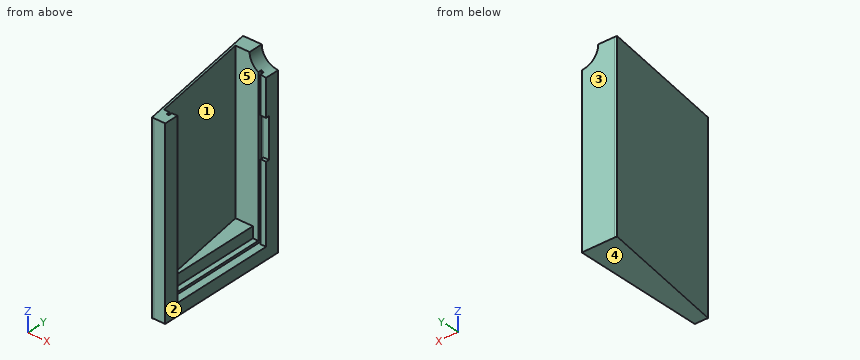
```python
from build123d import *

# Parameters (mm, degrees)
BOSS_EXTRUDE3_DEPTH = 40
SKETCH4_W           = 2
SKETCH4_H           = 142
CUT_EXTRUDE1_DEPTH  = 3
SKETCH5_W           = 2
SKETCH5_H           = 98
CUT_EXTRUDE2_DEPTH  = 3
SKETCH6_W           = 2
SKETCH6_H           = 145
CUT_EXTRUDE3_DEPTH  = 3
CUT_EXTRUDE4_DEPTH  = 228
SKETCH8_W           = 165
SKETCH8_H           = 122.641754717
BOSS_EXTRUDE5_DEPTH = 2
SKETCH11_W          = 2
SKETCH11_H          = 0.3
CUT_EXTRUDE5_DEPTH  = 145
SKETCH12_W          = 2
SKETCH12_H          = 0.3
CUT_EXTRUDE6_DEPTH  = 145
SKETCH16_W          = 2
SKETCH16_H          = 101.6
CUT_EXTRUDE7_DEPTH  = 154
SKETCH17_W          = 10
SKETCH17_H          = 95
CUT_EXTRUDE9_DEPTH  = 12
SKETCH18_W          = 5
SKETCH18_H          = 5
CUT_EXTRUDE10_DEPTH = 56
SKETCH19_W          = 36
SKETCH19_H          = 3
CUT_EXTRUDE11_DEPTH = 6
CUT_EXTRUDE13_DEPTH = 27
SKETCH22_W          = 2
SKETCH22_H          = 95
CUT_EXTRUDE22_DEPTH = 5
CUT_EXTRUDE23_DEPTH = 154


with BuildPart() as part:
    # Sketch2 → Boss-Extrude3 (new body)
    with BuildSketch(Plane(origin=(0, 0, 0), x_dir=(0, 0, -1), z_dir=(1, 0, 0))):
        Polygon((-34.1264251, 9.12857495), (-34.1264251, -3.87142505), (130.8735749, -3.87142505), (130.8735749, 117.12857495), (-34.1264251, 117.12857495), (-34.1264251, 104.12857495), (107.8735749, 104.12857495), (107.8735749, 9.12857495), align=None)
    extrude(amount=BOSS_EXTRUDE3_DEPTH)

    # Sketch4 → Cut-Extrude1 (cut)
    with BuildSketch(Plane.XZ.offset(-104.12857495)):
        with Locations((34, -36.8735749)):
            Rectangle(SKETCH4_W, SKETCH4_H)
    extrude(amount=-CUT_EXTRUDE1_DEPTH, mode=Mode.SUBTRACT)

    # Sketch5 → Cut-Extrude2 (cut)
    with BuildSketch(Plane.XY.offset(-107.8735749)):
        with Locations((34, 58.12857495)):
            Rectangle(SKETCH5_W, SKETCH5_H)
    extrude(amount=-CUT_EXTRUDE2_DEPTH, mode=Mode.SUBTRACT)

    # Sketch6 → Cut-Extrude3 (cut)
    with BuildSketch(Plane(origin=(0, 9.12857495, 0), x_dir=(1, 0, 0), z_dir=(0, 1, 0))):
        with Locations((34, 38.3735749)):
            Rectangle(SKETCH6_W, SKETCH6_H)
    extrude(amount=-CUT_EXTRUDE3_DEPTH, mode=Mode.SUBTRACT)

    # Sketch7 → Cut-Extrude4 (cut)
    with BuildSketch(Plane(origin=(0, 0, -130.8735749), x_dir=(-1, 0, 0), z_dir=(0, 0, -1))):
        Polygon((0, 117.12857495), (0, -3.87142505), (-30, -3.87142505), (-10, 117.12857495), align=None)
    extrude(amount=-CUT_EXTRUDE4_DEPTH, mode=Mode.SUBTRACT)

    # Sketch8 → Boss-Extrude5 (add)
    with BuildSketch(Plane(origin=(28.579293357, 4.723850142, 0), x_dir=(0, 0, 1), z_dir=(-0.986613411390535, -0.16307659692405535, 0))):
        with Locations((-48.3735749, 52.608979576)):
            Rectangle(SKETCH8_W, SKETCH8_H)
    extrude(amount=BOSS_EXTRUDE5_DEPTH)

    # Sketch11 → Cut-Extrude5 (cut)
    with BuildSketch(Plane.XY.offset(34.1264251)):
        with Locations((34, 107.27857495)):
            Rectangle(SKETCH11_W, SKETCH11_H)
    extrude(amount=-CUT_EXTRUDE5_DEPTH, mode=Mode.SUBTRACT)

    # Sketch12 → Cut-Extrude6 (cut)
    with BuildSketch(Plane.XY.offset(34.1264251)):
        with Locations((34, 5.97857495)):
            Rectangle(SKETCH12_W, SKETCH12_H)
    extrude(amount=-CUT_EXTRUDE6_DEPTH, mode=Mode.SUBTRACT)

    # Sketch16 → Cut-Extrude7 (cut)
    with BuildSketch(Plane.XY.offset(34.1264251)):
        with Locations((34, 56.62857495)):
            Rectangle(SKETCH16_W, SKETCH16_H)
    extrude(amount=-CUT_EXTRUDE7_DEPTH, mode=Mode.SUBTRACT)

    # Sketch17 → Cut-Extrude9 (cut)
    with BuildSketch(Plane(origin=(40, 0, 0), x_dir=(0, 0, -1), z_dir=(1, 0, 0))):
        with Locations((112.8735749, 56.62857495)):
            Rectangle(SKETCH17_W, SKETCH17_H)
    extrude(amount=-CUT_EXTRUDE9_DEPTH, mode=Mode.SUBTRACT)

    # Sketch18 → Cut-Extrude10 (cut)
    with BuildSketch(Plane.XZ.offset(-104.12857495)):
        with Locations((30.5, 31.6264251)):
            Rectangle(SKETCH18_W, SKETCH18_H)
    extrude(amount=-CUT_EXTRUDE10_DEPTH, mode=Mode.SUBTRACT)

    # Sketch19 → Cut-Extrude11 (cut)
    with BuildSketch(Plane(origin=(40, 0, 0), x_dir=(0, 0, -1), z_dir=(1, 0, 0))):
        with Locations((31.8735749, 105.62857495)):
            Rectangle(SKETCH19_W, SKETCH19_H)
    extrude(amount=-CUT_EXTRUDE11_DEPTH, mode=Mode.SUBTRACT)

    # Sketch20 → Cut-Extrude13 (cut)
    with BuildSketch(Plane(origin=(0, 117.12857495, 0), x_dir=(1, 0, 0), z_dir=(0, 1, 0))):
        with BuildLine():
            Line((33, -34.1264251), (40, -34.1264251))
            Line((40, -34.1264251), (40, -19.1264251))
            ThreePointArc((40, -19.1264251), (29.393398282, -23.519823382), (25, -34.1264251))
            Line((25, -34.1264251), (28, -34.1264251))
            Line((28, -34.1264251), (28, -29.1264251))
            Line((28, -29.1264251), (33, -29.1264251))
            Line((33, -29.1264251), (33, -34.1264251))
        make_face()
    extrude(amount=-CUT_EXTRUDE13_DEPTH, mode=Mode.SUBTRACT)

    # Sketch22 → Cut-Extrude22 (cut)
    with BuildSketch(Plane(origin=(40, 0, 0), x_dir=(0, 0, -1), z_dir=(1, 0, 0))):
        with Locations((118.8735749, 56.62857495)):
            Rectangle(SKETCH22_W, SKETCH22_H)
    extrude(amount=-CUT_EXTRUDE22_DEPTH, mode=Mode.SUBTRACT)

    # Sketch23 → Cut-Extrude23 (cut)
    with BuildSketch(Plane.XY.offset(34.1264251)):
        Polygon((33, 5.82857495), (35, 5.82857495), (35.1, 5.82857495), (35.1, 107.42857495), (35, 107.42857495), (33, 107.42857495), (32.9, 107.42857495), (32.9, 5.82857495), align=None)
    extrude(amount=-CUT_EXTRUDE23_DEPTH, mode=Mode.SUBTRACT)


solid = part.part
```
Could you check a few things on this model? Use its own coordinates, in mm. Face numbers are marked on the shaded views. A direction names the side the tool comes from. Give positions to 0.01 mm unless a question says otherwise; leave off trailing zeros. Order: outer loops, then holes, each group sorted by start corner. A loop starts at its lowest first (then second) coordinate and runs counter-clockwise, first axis right, second up.
Q1. Suppose I cut it at D-D, the plane z = -110. Write out the boundary of the cut face in (x, y), and give its area (3 significant figures).
Q2. For the marked faces 4 and 5, which set-ups out of +Z, -Z, +X, -X, +Y, -Y let a thin tool reach every point of the face, with its end or its side?
Q3. We'd pull the mould along Y, two halves only. Please class the marked faces 1, 2 and 3: +Y half, -Y half, draft (parallel to the pull), parting line (faces both ways), or undercut.
Q4. I'm going to push flat-ended pins straight in: P1, Ø10, axis at x = 23.5, y = 93.5, coming from the +Z side; P2, Ø3, axis at y = 51, z = -112, coming from the +X side; P3, Ø6, axis at x = 27.5, z = -35.5, coming from the -Y side; P4, Ø0.7, axis at x = 33.5, z = -47.5, coming from the -Y side. Where does each tip first touch, or does it pass through?
Q5. Suppose I cut it at B-B, the plane y = 99. Write out the boundary of the cut face in (x, z).
Q6. Suppose I cut it at C-C, the plane x = 37.5. Write out the boundary of the cut face in (y, z).
Q7. If I drill on line 1 along Y through (x, z) = (33.5, -79); line 2 along Y through (x, z) = (38.5, 13); line 3 along Z through (x, y) = (36.5, 87.5), over which ranges is the centre line in solid material (lowest first)?
Q8. Suppose I cut it at A-A, the plane z = -74.5. Write out the boundary of the cut face in (x, y), and give its area (3 significant figures).
Solution:
1. outline: (8.03, 116.8) - (28.03, -4.2) - (30, -3.87) - (40, -3.87) - (40, 9.13) - (35.1, 9.13) - (35.1, 5.83) - (32.9, 5.83) - (32.9, 9.13) - (28, 9.13) - (28, 104.13) - (32.9, 104.13) - (32.9, 107.43) - (35.1, 107.43) - (35.1, 104.13) - (40, 104.13) - (40, 117.13) - (10, 117.13) - close
1. area: 1,510 mm2
2. face 4: -Z, +X, -X, +Y, -Y
2. face 5: +Z, +X
3. face 1: undercut
3. face 2: draft
3. face 3: +Y half
4. P1: stops at z = -107.87
4. P2: stops at x = 28
4. P3: stops at y = -4.2
4. P4: stops at y = -3.87
5. outline: (10.97, -130.87) - (40, -130.87) - (40, -119.87) - (32.9, -119.87) - (32.9, -117.87) - (28, -117.87) - (28, -107.87) - (13, -107.87) - (13, 34.13) - (10.97, 34.13) - close
6. outline: (-3.87, -130.87) - (117.13, -130.87) - (117.13, 19.34) - (104.13, 19.34) - (104.13, -13.87) - (107.13, -13.87) - (107.13, -49.87) - (104.13, -49.87) - (104.13, -119.87) - (9.13, -119.87) - (9.13, 34.13) - (-3.87, 34.13) - close
7. line 1: y = -3.87 to 5.83, 107.43 to 117.13
7. line 2: y = -3.87 to 9.13, 104.13 to 117.13
7. line 3: z = -130.87 to -119.87
8. outline: (8.03, 116.8) - (28.03, -4.2) - (30, -3.87) - (40, -3.87) - (40, 9.13) - (35.1, 9.13) - (35.1, 5.83) - (32.9, 5.83) - (32.9, 9.13) - (27.85, 9.13) - (12.15, 104.13) - (32.9, 104.13) - (32.9, 107.43) - (35.1, 107.43) - (35.1, 104.13) - (40, 104.13) - (40, 117.13) - (10, 117.13) - close
8. area: 751 mm2
